Build history of the part. All positions in model axes, mm. Face numbers are marked on the shaded views. A direction names the side the tool comes from. Round coordinates to 2 decimals unless told otherwise and drop trailing zeros. Write each loop counter-clockwise with the first axis right and the second up, starting at its lowest first coordinate (ties: lowest second). Pieces come first, ordered by that corner, then holes. Notation, with made-up numbers: M -21.5,22.5 L -15.5,22.5 A6 ccw -15.5,31.5 Z; hole C -28,-32 d8. An arc over 180 degrees is marked long. Use a Markdown table: item, result.
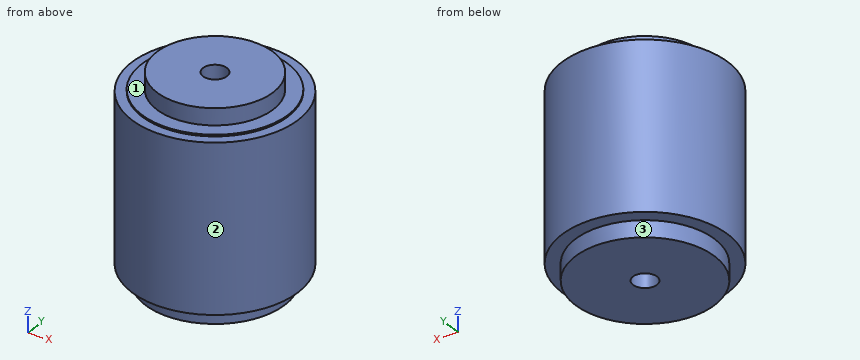
from build123d import *

# Parameters (mm, degrees)
F0_R     = 25
F0_R_2   = 3.6
F1_DEPTH = 50
F2_R     = 21
F2_R_2   = 3.6
F3_DEPTH = 5
F4_R     = 22
F4_R_2   = 3.6
F5_DEPTH = 0.5
F6_R     = 17.5
F6_R_2   = 3.6
F7_DEPTH = 5


with BuildPart() as f1:
    # F0 (on Top) → F1 (new body)
    with BuildSketch(Plane.XY):
        Circle(F0_R)
        Circle(F0_R_2, mode=Mode.SUBTRACT)
    extrude(amount=F1_DEPTH)

    # F2 (on face) → F3 (join)
    with BuildSketch(Plane(origin=(0, 0, 0), x_dir=(1, 0, 0), z_dir=(0, 0, -1))):
        Circle(F2_R)
        Circle(F2_R_2, mode=Mode.SUBTRACT)
    extrude(amount=F3_DEPTH)

    # F4 (on face) → F5 (join)
    with BuildSketch(Plane.XY.offset(50)):
        Circle(F4_R)
        Circle(F4_R_2, mode=Mode.SUBTRACT)
    extrude(amount=F5_DEPTH)

    # F6 (on face) → F7 (join)
    with BuildSketch(Plane.XY.offset(50.5)):
        Circle(F6_R)
        Circle(F6_R_2, mode=Mode.SUBTRACT)
    extrude(amount=F7_DEPTH)


solid = f1.part
Q1. Drop flat-ended pins along their axis: P1, Ø8, axis at x = -6, z = 25, coming from the -Y side; P2, Ø2, axis at y = 14, z = 10.5, coming from the +X side; P3, Ø3, axis at y = 2, z = 36, coming from the +X side (3 decimals). Give the stop position or say it passes through.
Response values:
| item | result |
|---|---|
| P1 | stops at y = -24.92 |
| P2 | stops at x = 21.35 |
| P3 | stops at x = 24.995 |
Q2. Cut at D-D on y = 12. Give the cut face in (x, z), and give its area (3 significant figures).
Response values:
| item | result |
|---|---|
| outline | M -21.93,0 L -17.23,0 L -17.23,-5 L 17.23,-5 L 17.23,0 L 21.93,0 L 21.93,50 L 18.44,50 L 18.44,50.5 L 12.74,50.5 L 12.74,55.5 L -12.74,55.5 L -12.74,50.5 L -18.44,50.5 L -18.44,50 L -21.93,50 Z |
| area | 2,510 mm2 |
Q3. Which spindle directions (+Z, -Z, +X, -X, +Y, -Y) get a long thin tool onto all of the face, cutting with end or side? Do the marked faces 1, 2 and 3. Say none if no direction does.
Response values:
| item | result |
|---|---|
| face 1 | +Z |
| face 2 | +Z, -Z |
| face 3 | -Z |
Q4. Cut at A-A on x = 0. Give the cut face in (y, z).
Response values:
| item | result |
|---|---|
| outline | M -25,0 L -21,0 L -21,-5 L -3.6,-5 L -3.6,55.5 L -17.5,55.5 L -17.5,50.5 L -22,50.5 L -22,50 L -25,50 Z; M 3.6,-5 L 21,-5 L 21,0 L 25,0 L 25,50 L 22,50 L 22,50.5 L 17.5,50.5 L 17.5,55.5 L 3.6,55.5 Z |
Q5. Drill centre lines: L1, parallel to Y at x = 0, z = 9; L2, parallel to X at y = -2, z = 16; L3, parallel to Z at x = -17, y = -15. Where is each one in solid material? Low to high.
Response values:
| item | result |
|---|---|
| L1 | y = -25 to -3.6, 3.6 to 25 |
| L2 | x = -24.92 to -2.99, 2.99 to 24.92 |
| L3 | z = 0 to 50 |
Q6. Cut at C-C on z = 37. Give the cut face in (x, y).
Response values:
| item | result |
|---|---|
| outline | C 0,0 d50; hole C 0,0 d7.2 |
